Geometry: final body of the model. Coordinates: model frame, mm. A direction names the side the tool comes from. Round coordinates to 2 decimals unless told otherwise and drop trailing zeros. Loops run counter-clockwise (first coordinate to the right, second up) from the corner with the lowest first, then second, coordinate; pieces in that order, holes last. Notation, with made-up numbers: (9.25, 56) -> (14.25, 56) arc R16 cw to (14.25, 66) -> close; hole circle Ø1 at (-23.5, -24.75). An arc over 180 degrees is marked (long way). Answer in a Markdown table with one row per item.
```python
from build123d import *

# Parameters (mm, degrees)
F0_R      = 25
F1_DEPTH  = 12.5
F2_R      = 5
F2_R_2    = 2.5
F3_DEPTH  = 50
F2_R_3    = 10
F4_DEPTH  = 40
F2_R_4    = 15
F5_DEPTH  = 30
F2_R_5    = 20
F6_DEPTH  = 20
F2_R_6    = 25
F7_DEPTH  = 10
F2_R_7    = 1.25
F8_DEPTH  = 60
F9_DEPTH  = 70
F10_R     = 12.5
F11_DEPTH = 75


with BuildPart() as f1:
    # F0 (on Front) → F1 (new body, symmetric)
    with BuildSketch(Plane.XZ):
        Circle(F0_R)
    extrude(amount=F1_DEPTH, both=True)

    # F2 (on face) → F3 (join)
    with BuildSketch(Plane.XZ.offset(12.5)):
        Circle(F2_R)
        Circle(F2_R_2, mode=Mode.SUBTRACT)
    extrude(amount=F3_DEPTH)

    # F2 (on face) → F4 (join)
    with BuildSketch(Plane.XZ.offset(12.5)):
        Circle(F2_R_3)
        Circle(F2_R, mode=Mode.SUBTRACT)
    extrude(amount=F4_DEPTH)

    # F2 (on face) → F5 (join)
    with BuildSketch(Plane.XZ.offset(12.5)):
        Circle(F2_R_4)
        Circle(F2_R_3, mode=Mode.SUBTRACT)
    extrude(amount=F5_DEPTH)

    # F2 (on face) → F6 (join)
    with BuildSketch(Plane.XZ.offset(12.5)):
        Circle(F2_R_5)
        Circle(F2_R_4, mode=Mode.SUBTRACT)
    extrude(amount=F6_DEPTH)

    # F2 (on face) → F7 (join)
    with BuildSketch(Plane.XZ.offset(12.5)):
        Circle(F2_R_6)
        Circle(F2_R_5, mode=Mode.SUBTRACT)
    extrude(amount=F7_DEPTH)

    # F2 (on face) → F8 (join)
    with BuildSketch(Plane.XZ.offset(12.5)):
        Circle(F2_R_2)
        Circle(F2_R_7, mode=Mode.SUBTRACT)
    extrude(amount=F8_DEPTH)

    # F2 (on face) → F9 (join)
    with BuildSketch(Plane.XZ.offset(12.5)):
        Circle(F2_R_7)
    extrude(amount=F9_DEPTH)

    # F10 (on face) → F11 (join)
    with BuildSketch(Plane(origin=(0, 12.5, 0), x_dir=(-1, 0, 0), z_dir=(0, 1, 0))):
        Circle(F10_R)
    extrude(amount=F11_DEPTH)


solid = f1.part
```
Item 1: Reachability of faces 4 (the face through (-11.923, 49.475, 3.755)), 5 (the face through (3, -42.5, -10)), 6 (the face through (0, 87.5, 0)) from +Z, -Z, +X, -X, +Y, -Y: full face, straight path, thin tool, end or side. Return the list, or none.
Answer:
| item | result |
|---|---|
| face 4 | +Y |
| face 5 | -Y |
| face 6 | +Z, -Z, +X, -X, +Y |
Item 2: Pin query (flat end, axial travel): pin 1 Ø20 at (x, z) = (-3.5, -10) entering from -Y; pin 2 Ø10 at (y, z) = (4.5, -19) entering from +X; pin 3 Ø5 at (x, z) = (-10.5, 13.5) entering from +Y; pin 4 Ø6 at (x, y) = (17.5, -20) entering from -Z. Return the tip coordinate at first contact, or that it passes through.
Answer:
| item | result |
|---|---|
| pin 1 | stops at y = -82.5 |
| pin 2 | stops at x = 20.71 |
| pin 3 | stops at y = 12.5 |
| pin 4 | stops at z = -20.37 |
Item 3: Draft query along Y for faces 1 (the face through (-11.5, 12.5, 5.9)), 2 (the face through (-11, -22.5, 17)), 3 (the face through (-1.08, -57.43, -4.88)). Return one class per face: pulls with the +Y half, pulls with the -Y half, needs draft (parallel to the pull), parting line crosses it, or undercut.
Answer:
| item | result |
|---|---|
| face 1 | pulls with the +Y half |
| face 2 | pulls with the -Y half |
| face 3 | needs draft |
Item 4: Cut plane A-A (y = 42). Output: boundary loops of the cut face in (x, z).
Answer:
| item | result |
|---|---|
| outline | circle Ø25 at (0, 0) |
Item 5: Cut plane C-C (y = -24.5). Output: boundary loops of the cut face in (x, z), then the cut area to 3 significant figures.
Answer:
| item | result |
|---|---|
| outline | circle Ø40 at (0, 0) |
| area | 1,260 mm² |
Item 6: Line query: probe 1 along Y at (x, z) = (-11.5, -15); probe 2 along Y at (x, z) = (-4.5, -5); probe 3 along X at (y, z) = (-23, -1). Output: solid intervals per line, ascending. Write a range as [from, to].
Answer:
| item | result |
|---|---|
| probe 1 | y = [-32.5, 12.5] |
| probe 2 | y = [-52.5, 87.5] |
| probe 3 | x = [-19.97, 19.97] |
Item 7: Cut plane B-B (x = -16.5). Output: boundary loops of the cut face in (y, z), then the cut area to 3 significant figures.
Answer:
| item | result |
|---|---|
| outline | (-32.5, -11.3) -> (-22.5, -11.3) -> (-22.5, -18.78) -> (12.5, -18.78) -> (12.5, 18.78) -> (-22.5, 18.78) -> (-22.5, 11.3) -> (-32.5, 11.3) -> close |
| area | 1,540 mm² |
